Geometry: final body of the model. Coordinates: model frame, mm. A direction names the side the tool comes from. Give positions to 0.01 mm unless a question says otherwise; leave off trailing zeros. Order: outer loops, then holes, each group sorted by start corner. A loop starts at its lowest first (then second) coordinate and runs counter-clockwise, first axis right, second up. Notation, with made-up numbers: (35, 10.25) -> (59, 10.25) arc R32 ccw to (59, 43.25) -> close; hole circle Ø7 at (4.25, 32.25). An arc over 180 degrees is marked (long way). One line per question, with ' | ' between items.
from build123d import *

# Parameters (mm, degrees)
F0_W     = 50
F0_H     = 20
F1_DEPTH = 2.5
F2_R     = 2
F3_DEPTH = 5.001
F4_R     = 1.5
F5_DEPTH = 5


with BuildPart() as f1:
    # F0 (on Top) → F1 (new body, symmetric)
    with BuildSketch(Plane.XY):
        with Locations((1.897323, 0)):
            Rectangle(F0_W, F0_H)
    extrude(amount=F1_DEPTH, both=True)

    # F2 (on face) → F3 (cut, through all)
    with BuildSketch(Plane.XY.offset(2.5)):
        with Locations((22.897323, 0)):
            Circle(F2_R)
    extrude(amount=-F3_DEPTH, mode=Mode.SUBTRACT)

    # F4 (on face) → F5 (cut)
    with BuildSketch(Plane.YZ.offset(26.897323)):
        Circle(F4_R)
    extrude(amount=-F5_DEPTH, mode=Mode.SUBTRACT)


solid = f1.part
1) Section A-A on y = 0. Return loops of the section in (x, z).
Check result:
outline: (-23.1, -2.5) -> (20.9, -2.5) -> (20.9, 2.5) -> (-23.1, 2.5) -> close; (24.9, -2.5) -> (26.9, -2.5) -> (26.9, -1.5) -> (24.9, -1.5) -> close; (24.9, 1.5) -> (26.9, 1.5) -> (26.9, 2.5) -> (24.9, 2.5) -> close
2) Material intervals for probe 1 along Y at (x, z) = (26, 0); probe 2 along Z at (x, y) = (25.35, 0); probe 3 along X at (y, z) = (1, -0.85), sorted ascending. Write a range as from..to.
Check result:
probe 1: y = -10..-1.5, 1.5..10 | probe 2: z = -2.5..-1.5, 1.5..2.5 | probe 3: x = -23.1..21.17
3) Section B-B on x = 23.5. Return loops of the section in (y, z), plus the area to 3 significant figures.
Check result:
outline: (-10, -2.5) -> (-1.91, -2.5) -> (-1.91, 2.5) -> (-10, 2.5) -> close; (1.91, -2.5) -> (10, -2.5) -> (10, 2.5) -> (1.91, 2.5) -> close | area: 80.9 mm^2
4) Set-up query: faces 1 (the flat face through (2, 0, 2.5)), 2 (the cylindrical face through (25.875, 1.386, -0.575)). Return all of +Z, -Z, +X, -X, +Y, -Y with unobstructed straight access to the full face (end or side cutting, diameter ignored); none if empty.
Check result:
face 1: +Z, +X, -X, +Y, -Y | face 2: +X
5) Contact query for a flat-ended pin moving along its axis: pin 1 Ø2.5 at (x, y) = (22.9, 0) entering from +Z. Output: stop coordinate, or through.
Check result:
pin 1: passes through
6) Pull-direction query (X, two-part tool) for faces 3 (the flat face through (-23.103, 0, 0)), 4 (the flat face through (26.897, 0, 2)), 5 (the cylindrical face through (20.9, 0.1, 0)), 6 (the flat face through (2, -10, 0)); classes: +X half, -X half, draft (parallel to the pull), parting line (faces both ways), or undercut.
Check result:
face 3: -X half | face 4: +X half | face 5: undercut | face 6: draft
7) Section C-C on z = 0. Return loops of the section in (x, y), plus the area to 3 significant figures.
Check result:
outline: (-23.1, -10) -> (26.9, -10) -> (26.9, -1.5) -> (24.22, -1.5) arc R2 cw (long way) to (24.22, 1.5) -> (26.9, 1.5) -> (26.9, 10) -> (-23.1, 10) -> close | area: 981 mm^2
